Input: part model. Units: mm. Frame: model coordinates. Face numbers are marked on the shaded views. A direction names the side the tool comes from. Round coordinates to 2 decimals unless told otherwise and drop trailing zeros. Loops run counter-clockwise (first coordinate to the right, second up) from the corner with the lowest first, then second, coordinate; pieces in that order, holes last. Notation, with made-up numbers: (4.5, 29) -> (12.5, 29) arc R15 cw to (12.5, 53) -> close; hole circle Ø1 at (12.5, -21.5). An arc over 180 degrees is marked (long way). Answer in a Markdown table with one row per item. Add a question column.
Q1. Section A-A, the plane z = 12.5. Output: boundary loops of the cut face in (x, y).
Q2. Section D-D, the plane x = 8. Output: boundary loops of the cut face in (y, z), and give its area (3 significant figures).
Q3. Ray query, L1, parallel to X at y = 3.5, z = 5.5; L2, parallel to Y at x = -14.5, z = 13.25; L3, parallel to Z at x = 8, y = 6. Return the intervals inside material, ascending. Write a range as from..to.
Q4. Section B-B, the plane x = 21. Output: boundary loops of the cut face in (y, z), and give its area (3 significant figures).
Q5. Section C-C, the plane y = 32. Output: boundary loops of the cut face in (x, z), and give its area (3 significant figures).
Q6. Mould query, pull axis X, two halves, no side actions, for the marked faces 6, 7 and 8. Classes: pulls with the +X half, pulls with the -X half, needs draft (parallel to the pull), parting line crosses it, or undercut.
Q7. Pin query (flat end, axial travel): pin 1 (5.5 mm diameter, centred on y = 3, z = 7, fed in from +X); pin 2 (5.5 mm diameter, centred on y = -2, z = 9, fed in from -X); pin 3 (1.4 mm diameter, centred on x = -21, z = 6.5, fed in from +Y). Return the tip coordinate at first contact, or that it passes through.
Q8. Reachability of the marked faces 1, 2, 3, 4 and 5 from +Z, -Z, +X, -X, +Y, -Y: full face, straight path, thin tool, end or side. Return the list, or none.
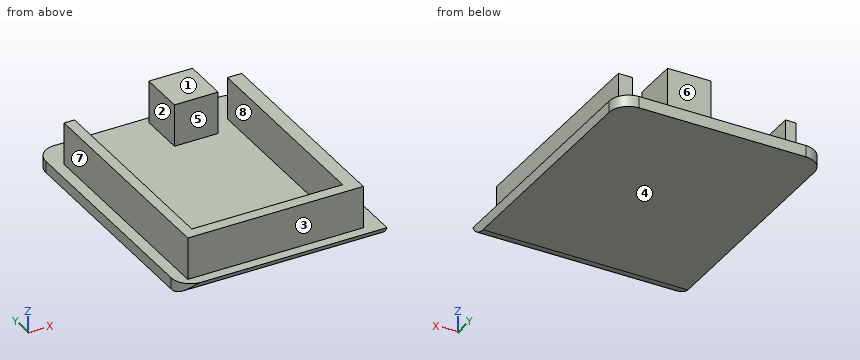
```python
from build123d import *

# Parameters (mm, degrees)
F1_DEPTH    = 14
F0_W        = 11.3450561184
F0_H        = 11.8383169174
F0_W_2      = 53.3
F0_H_2      = 68
F2_DEPTH    = 3
F3_T1_DEPTH = 28
F3_T3_DEPTH = 76.2128784748


# Not quite as in the source:
# - a fillet or chamfer that OpenCascade refuses, or shapes differently, is made with other operations: its cross-section is extruded or revolved along the edge and cut away or added


with BuildPart() as f1:
    # F0 (on Top) → F1 (new body)
    with BuildSketch(Plane.XY):
        Polygon((-20.2707853168, 36.2087599933), (-22.9837335646, 36.2087599933), (-22.9837335646, -18.0502012372), (-22.9837335646, -21.0097823292), (-20.2707853168, -21.0097823292), (18.9436431974, -21.0097823292), (22.6431209594, -21.0097823292), (22.6431209594, -18.0502012372), (22.6431209594, 35.2222323418), (18.9436431974, 35.2222323418), (18.9436431974, -18.0502012372), (-20.2707853168, -18.0502012372), align=None)
    extrude(amount=F1_DEPTH)



with BuildPart() as f1b:
    # F0 (on Top) → F1, piece 2 (new body)
    with BuildSketch(Plane.XY):
        with Locations((8.338484331, 36.7020219564)):
            Rectangle(F0_W, F0_H)
    extrude(amount=F1_DEPTH)


with BuildPart() as f1_1:
    add(f1.part)

    add(f1b.part)  # F2 merges F1b
    # F0 (on Top) → F2 (join)
    with BuildSketch(Plane.XY):
        with Locations((0.7177972624, 10.4120122269)):
            Rectangle(F0_W_2, F0_H_2)
        Polygon((-22.9837335646, -18.0502012372), (-22.9837335646, 36.2087599933), (-20.2707853168, 36.2087599933), (-20.2707853168, -18.0502012372), (18.9436431974, -18.0502012372), (18.9436431974, 35.2222323418), (22.6431209594, 35.2222323418), (22.6431209594, -18.0502012372), (22.6431209594, -21.0097823292), (18.9436431974, -21.0097823292), (-20.2707853168, -21.0097823292), (-22.9837335646, -21.0097823292), align=None, mode=Mode.SUBTRACT)
        with Locations((8.338484331, 36.7020219564)):
            Rectangle(F0_W, F0_H, mode=Mode.SUBTRACT)
    extrude(amount=F2_DEPTH)

    # F3: fillet of radius 5 on 4 edges, made by hand

    # F3_s2 → F3_t1 (cut)
    with BuildSketch(Plane.XY.offset(-12.5)):
        with BuildLine():
            ThreePointArc((-20.9322027376, 44.4120122269), (-24.4677366436, 42.9475461328), (-25.9322027376, 39.4120122269))
            Line((-25.9322027376, 39.4120122269), (-25.9322027376, 44.4120122269))
            Line((-25.9322027376, 44.4120122269), (-20.9322027376, 44.4120122269))
        make_face()
        with BuildLine():
            ThreePointArc((-25.9322027376, -18.5879877731), (-24.4677366436, -22.1235216791), (-20.9322027376, -23.5879877731))
            Line((-20.9322027376, -23.5879877731), (-25.9322027376, -23.5879877731))
            Line((-25.9322027376, -23.5879877731), (-25.9322027376, -18.5879877731))
        make_face()
        with BuildLine():
            ThreePointArc((22.3677972624, 44.4120122269), (25.9033311683, 42.9475461328), (27.3677972624, 39.4120122269))
            Line((27.3677972624, 39.4120122269), (27.3677972624, 44.4120122269))
            Line((27.3677972624, 44.4120122269), (22.3677972624, 44.4120122269))
        make_face()
    extrude(amount=F3_T1_DEPTH, mode=Mode.SUBTRACT)

    # F3_s4 → F3_t3 (cut)
    with BuildSketch(Plane.YZ.offset(-37.388641975)):
        with BuildLine():
            ThreePointArc((-23.5879877731, 3), (-21.7440248657, 0.8166998673), (-19.0054120782, 0))
            Line((-19.0054120782, 0), (-23.5879877731, 0))
            Line((-23.5879877731, 0), (-23.5879877731, 3))
        make_face()
    extrude(amount=F3_T3_DEPTH, mode=Mode.SUBTRACT)


solid = f1_1.part
```
Answer block:
| question | item | result |
|---|---|---|
| 1 | outline | (-22.98, -21.01) -> (22.64, -21.01) -> (22.64, 35.22) -> (18.94, 35.22) -> (18.94, -18.05) -> (-20.27, -18.05) -> (-20.27, 36.21) -> (-22.98, 36.21) -> close; (2.67, 30.78) -> (14.01, 30.78) -> (14.01, 42.62) -> (2.67, 42.62) -> close |
| 2 | outline | (-23.59, 3) arc R5 ccw to (-19.01, 0) -> (44.41, 0) -> (44.41, 3) -> (42.62, 3) -> (42.62, 14) -> (30.78, 14) -> (30.78, 3) -> (-18.05, 3) -> (-18.05, 14) -> (-21.01, 14) -> (-21.01, 3) -> close |
| 2 | area | 363 mm^2 |
| 3 | L1 | -22.98..-20.27, 18.94..22.64 |
| 3 | L2 | -21.01..-18.05 |
| 3 | L3 | 0..3 |
| 4 | outline | (-23.59, 3) arc R5 ccw to (-19.01, 0) -> (44.41, 0) -> (44.41, 3) -> (35.22, 3) -> (35.22, 14) -> (-21.01, 14) -> (-21.01, 3) -> close |
| 4 | area | 819 mm^2 |
| 5 | outline | (-25.93, 0) -> (27.37, 0) -> (27.37, 3) -> (22.64, 3) -> (22.64, 14) -> (18.94, 14) -> (18.94, 3) -> (14.01, 3) -> (14.01, 14) -> (2.67, 14) -> (2.67, 3) -> (-20.27, 3) -> (-20.27, 14) -> (-22.98, 14) -> (-22.98, 3) -> (-25.93, 3) -> close |
| 5 | area | 355 mm^2 |
| 6 | face 6 | needs draft |
| 6 | face 7 | pulls with the -X half |
| 6 | face 8 | undercut |
| 7 | pin 1 | x = 22.64 |
| 7 | pin 2 | x = -22.98 |
| 7 | pin 3 | y = 36.21 |
| 8 | face 1 | +Z, +X, -X, +Y, -Y |
| 8 | face 2 | +Z, +Y |
| 8 | face 3 | +Z, +X, -X, -Y |
| 8 | face 4 | -Z, +X, -X, +Y, -Y |
| 8 | face 5 | +Z |
